Geometry check sheet. Reference: the model listing, model coordinates, mm. A direction names the side the tool comes from. Round coordinates to 2 decimals unless told otherwise and drop trailing zeros. Order: outer loops, then holes, each group sorted by start corner. A loop starts at its lowest first (then second) coordinate and runs counter-clockwise, first axis right, second up. Notation, with made-up numbers: (39.25, 34) - (87.25, 34) arc R17 cw to (87.25, 60) - close; hole circle Ø8 at (-24, 38). An arc over 180 degrees is marked (long way). Write each question's results on one line, items separated by ' | '.
```python
from build123d import *

# Parameters (mm, degrees)
F0_W      = 127
F0_H      = 203.2
F1_DEPTH  = 12.7
F2_W      = 127
F2_H      = 281.5760534146
F3_DEPTH  = 12.7
F4_R      = 3.6195
F5_DEPTH  = 12.7
F6_R      = 3.6195
F7_DEPTH  = 12.7
F8_R      = 3.6195
F9_DEPTH  = 12.7
F10_R     = 3.6195
F11_DEPTH = 12.7


with BuildPart() as f1:
    # F0 (on Front) → F1 (new body)
    with BuildSketch(Plane.XZ):
        with Locations((63.5, 101.6)):
            Rectangle(F0_W, F0_H)
    extrude(amount=-F1_DEPTH)

    # F2 (on face) → F3 (join)
    with BuildSketch(Plane.XY.offset(203.2)):
        with Locations((63.5, -140.7880267073)):
            Rectangle(F2_W, F2_H)
    extrude(amount=-F3_DEPTH)

    # F4 (on face) → F5 (cut)
    with BuildSketch(Plane.XZ):
        with Locations((92.6856547594, 64.833432436)):
            Circle(F4_R)
    extrude(amount=-F5_DEPTH, mode=Mode.SUBTRACT)

    # F6 (on face) → F7 (cut)
    with BuildSketch(Plane.XZ):
        with Locations((92.9278507829, 134.2175006866)):
            Circle(F6_R)
    extrude(amount=-F7_DEPTH, mode=Mode.SUBTRACT)

    # F8 (on face) → F9 (cut)
    with BuildSketch(Plane.XZ):
        with Locations((23.0624806136, 64.2787441611)):
            Circle(F8_R)
    extrude(amount=-F9_DEPTH, mode=Mode.SUBTRACT)

    # F10 (on face) → F11 (cut)
    with BuildSketch(Plane.XZ):
        with Locations((23.0022147298, 134.1594159603)):
            Circle(F10_R)
    extrude(amount=-F11_DEPTH, mode=Mode.SUBTRACT)


solid = f1.part
```
(1) Section check B-B (x = 56). Record the cut outline in (y, z), then the cut area to 3 significant figures.
Answers follow:
outline: (-281.58, 190.5) - (0, 190.5) - (0, 0) - (12.7, 0) - (12.7, 203.2) - (-281.58, 203.2) - close | area: 6,160 mm²
(2) Depth check by flat-ended pin: pin 1 Ø9.5 at (x, z) = (92.69, 64.83) entering from -Y; pin 2 Ø10 at (x, y) = (32, -136) entering from -Z. Enter the tip coordinate at first touch or a pass-through.
Answers follow:
pin 1: y = 0 | pin 2: z = 190.5
(3) Section check C-C (z = 15). Record the cut outline in (x, y).
Answers follow:
outline: (0, 0) - (127, 0) - (127, 12.7) - (0, 12.7) - close
(4) Access from +Z, -Z, +X, -X, +Y, -Y to the whole of each face (thin tool, end or side, straight path). Record for faces 4 (the face through (63, 0, 97)), 5 (the face through (22.278, 6.261, 60.745)).
Answers follow:
face 4: -Z, +X, -X, -Y | face 5: +Y, -Y
(5) Draft check along Z on faces 1 (the face through (94.87, 6.26, 137.27)), 2 (the face through (63, 12.7, 103)), 3 (the face through (63, 6, 0)). Enter one of: released by +Z, released by -Z, zero draft, split by the parting line, or undercut.
Answers follow:
face 1: undercut | face 2: zero draft | face 3: released by -Z
(6) Section check A-A (y = -105). Record the cut outline in (x, z).
Answers follow:
outline: (0, 190.5) - (127, 190.5) - (127, 203.2) - (0, 203.2) - close
(7) Material ranges on line 1 (Z direction, x = 31, y = -151.5); line 2 (Y direction, x = 12.5, z = 79), recorded low to high.
Answers follow:
line 1: 190.5 to 203.2 | line 2: 0 to 12.7
